Verification items for the finished model (mm, model axes). A direction names the side the tool comes from. Round coordinates to 2 decimals unless told otherwise and drop trailing zeros. Write each loop counter-clockwise with the first axis right and the second up, starting at its lowest first coordinate (ties: lowest second). Pieces come first, ordered by that corner, then holes. Notation, with made-up numbers: M 39.5,-23.75 L 72.5,-23.75 A15 cw 72.5,-12.75 Z; hole C 48,-8 d4. An arc over 180 degrees is marked long. One line per question, with ' | ' between items.
from build123d import *

# Parameters (mm, degrees)
SKETCH1_W           = 4.7625
SKETCH1_H           = 50
SKETCH1_W_2         = 28.575
BOSS_EXTRUDE1_DEPTH = 4.7625
SKETCH1_3_W         = 4.7625
SKETCH1_3_H         = 50
BOSS_EXTRUDE2_DEPTH = 31.75
SKETCH3_R           = 4
CUT_EXTRUDE1_DEPTH  = 39.1
FILLET1_R           = 6.35
FILLET2_R           = 4.7625


with BuildPart() as part:
    # Sketch1 → Boss-Extrude1 (new body)
    with BuildSketch(Plane(origin=(0, 0, 0), x_dir=(1, 0, 0), z_dir=(0, 1, 0))):
        with Locations((-16.66875, 0)):
            Rectangle(SKETCH1_W, SKETCH1_H)
        Rectangle(SKETCH1_W_2, SKETCH1_H)
        with Locations((16.66875, 0)):
            Rectangle(SKETCH1_W, SKETCH1_H)
    extrude(amount=BOSS_EXTRUDE1_DEPTH)

    # Sketch1<3> → Boss-Extrude2 (add)
    with BuildSketch(Plane(origin=(0, 0, 0), x_dir=(1, 0, 0), z_dir=(0, 1, 0))):
        with Locations((-16.66875, 0)):
            Rectangle(SKETCH1_3_W, SKETCH1_3_H)
        with Locations((16.66875, 0)):
            Rectangle(SKETCH1_3_W, SKETCH1_3_H)
    extrude(amount=-BOSS_EXTRUDE2_DEPTH)

    # Sketch3 → Cut-Extrude1 (cut, through all)
    with BuildSketch(Plane(origin=(19.05, 0, 0), x_dir=(0, 0, -1), z_dir=(1, 0, 0))):
        Polygon((25, -31.75), (25, 0), (-12.3, -31.75), align=None)
        Polygon((-15.475, 0), (-15.475, 4.7625), (-25, 4.7625), (-25, 0), (-25, -14.247596398), align=None)
        with Locations((-16.745, -20.6375)):
            Circle(SKETCH3_R)
    extrude(amount=-CUT_EXTRUDE1_DEPTH, mode=Mode.SUBTRACT)

    # Fillet1
    fillet1_edges = [part.edges().sort_by_distance(p)[0] for p in [
        (-16.66875, -31.75, 25),
        (16.66875, -31.75, 25),
        (16.66875, -31.75, 12.3),
        (-16.66875, -31.75, 12.3),
        (16.66875, -14.247596398, 25),
        (-16.66875, -14.247596398, 25),
    ]]
    fillet(fillet1_edges, radius=FILLET1_R)

    # Fillet2
    fillet2_edges = [part.edges().sort_by_distance(p)[0] for p in [
        (14.2875, 0, -4.7625),
        (-14.2875, 0, -4.7625),
    ]]
    fillet(fillet2_edges, radius=FILLET2_R)


solid = part.part
1. Tool access check on faces 1 (the face through (17, -31.75, 17)), 2 (the face through (14.288, -15, 8)). Record the directions out of +Z, -Z, +X, -X, +Y, -Y that give a thin tool (end or side, any length) a straight path to the whole face; none if there is none.
Results:
face 1: +Z, -Z, +X, -X, -Y | face 2: +Z, -Z, -Y
2. Mould release check, pull along X, two halves, no side actions. Record for faces 3 (the face through (-19.05, -9, 6)), 4 (the face through (16.471, -14.906, -7.488)), 5 (the face through (-14.288, -15, 8)): pulls with the +X half, pulls with the -X half, needs draft (parallel to the pull), parting line crosses it, or undercut.
Results:
face 3: pulls with the -X half | face 4: needs draft | face 5: undercut
3. Thickness scan on line 1 (X direction, y = -9, z = -12); line 2 (Y direction, x = 3.5, z = -0.5). Record the ranges inside material, lowest first.
Results:
line 1: x = -19.05 to -14.29, 14.29 to 19.05 | line 2: y = 0 to 4.76
4. Go/stop test with flat-tipped pins: P1, Ø9.5, axis at x = -3.5, z = -10, coming from the -Y side; P2, Ø2.5, axis at x = -3.5, y = 3, coming from the +Z side (3 decimals). Record where each tip stops, or that it passes through.
Results:
P1: stops at y = 0 | P2: stops at z = 15.475
5. Section check A-A, the plane y = -10.5. Record the cut outline in (x, z), then the cut area to 3 significant figures.
Results:
outline: M -19.05,-12.66 L -14.29,-12.66 L -14.29,22.49 L -19.05,22.49 Z; M 14.29,-12.66 L 19.05,-12.66 L 19.05,22.49 L 14.29,22.49 Z | area: 335 mm2
6. Section check B-B, the plane z = 20. Record the cut outline in (x, y).
Results:
outline: M -19.05,-31.6 L -14.29,-31.6 L -14.29,-22.96 L -19.05,-22.96 Z; M -19.05,-18.31 L -14.29,-18.31 L -14.29,-6.77 L -19.05,-6.77 Z; M 14.29,-31.6 L 19.05,-31.6 L 19.05,-22.96 L 14.29,-22.96 Z; M 14.29,-18.31 L 19.05,-18.31 L 19.05,-6.77 L 14.29,-6.77 Z
7. Section check C-C, the plane x = -2. Record the cut outline in (y, z) (1 decimal), then the cut area to 3 significant figures.
Results:
outline: M 0,-25 L 4.8,-25 L 4.8,15.5 L 0,15.5 Z | area: 193 mm2
